```python
from build123d import *

# Parameters (mm, degrees)
SKETCH1_R           = 1.7526
BOSS_EXTRUDE1_DEPTH = 3


with BuildPart() as part:
    # Sketch1 → Boss-Extrude1 (new body)
    with BuildSketch(Plane.XY):
        with BuildLine():
            Line((-68.050090825, 31.75), (111.125, 31.75))
            Line((111.125, 31.75), (114.475, 31.75))
            Line((114.475, 31.75), (114.475, 19.05))
            Line((114.475, 19.05), (111.3, 19.05))
            Line((111.3, 19.05), (111.3, -6.35))
            Line((111.3, -6.35), (114.3, -6.35))
            Line((114.3, -6.35), (114.3, -18.229405084))
            Line((114.3, -18.229405084), (114.3, -19.870594916))
            Line((114.3, -19.870594916), (114.3, -31.75))
            Line((114.3, -31.75), (111.125, -31.75))
            Line((111.125, -31.75), (102.87, -31.75))
            Line((102.87, -31.75), (102.87, -34.75))
            Line((102.87, -34.75), (90.17, -34.75))
            Line((90.17, -34.75), (90.17, -31.75))
            Line((90.17, -31.75), (88.19515, -31.75))
            Line((88.19515, -31.75), (77.9653, -31.75))
            Line((77.9653, -31.75), (77.9653, -26.67))
            Line((77.9653, -26.67), (80.3275, -26.67))
            Line((80.3275, -26.67), (80.3275, -21.59))
            Line((80.3275, -21.59), (72.0725, -21.59))
            Line((72.0725, -21.59), (72.0725, -26.67))
            Line((72.0725, -26.67), (74.4347, -26.67))
            Line((74.4347, -26.67), (74.4347, -31.75))
            Line((74.4347, -31.75), (27.1653, -31.75))
            Line((27.1653, -31.75), (27.1653, -26.67))
            Line((27.1653, -26.67), (29.5275, -26.67))
            Line((29.5275, -26.67), (29.5275, -21.59))
            Line((29.5275, -21.59), (21.2725, -21.59))
            Line((21.2725, -21.59), (21.2725, -26.67))
            Line((21.2725, -26.67), (23.6347, -26.67))
            Line((23.6347, -26.67), (23.6347, -31.75))
            Line((23.6347, -31.75), (9.525, -31.75))
            Line((9.525, -31.75), (9.525, -34.75))
            Line((9.525, -34.75), (-9.525, -34.75))
            Line((-9.525, -34.75), (-9.525, -31.75))
            Line((-9.525, -31.75), (-23.6347, -31.75))
            Line((-23.6347, -31.75), (-23.6347, -26.67))
            Line((-23.6347, -26.67), (-21.2725, -26.67))
            Line((-21.2725, -26.67), (-21.2725, -21.59))
            Line((-21.2725, -21.59), (-29.5275, -21.59))
            Line((-29.5275, -21.59), (-29.5275, -26.67))
            Line((-29.5275, -26.67), (-27.1653, -26.67))
            Line((-27.1653, -26.67), (-27.1653, -31.75))
            Line((-27.1653, -31.75), (-41.275, -31.75))
            Line((-41.275, -31.75), (-41.275, -34.75))
            Line((-41.275, -34.75), (-60.325, -34.75))
            Line((-60.325, -34.75), (-60.325, -31.75))
            Line((-60.325, -31.75), (-74.4347, -31.75))
            Line((-74.4347, -31.75), (-74.4347, -26.67))
            Line((-74.4347, -26.67), (-72.0725, -26.67))
            Line((-72.0725, -26.67), (-72.0725, -21.59))
            Line((-72.0725, -21.59), (-80.3275, -21.59))
            Line((-80.3275, -21.59), (-80.3275, -26.67))
            Line((-80.3275, -26.67), (-77.9653, -26.67))
            Line((-77.9653, -26.67), (-77.9653, -31.75))
            Line((-77.9653, -31.75), (-114.3, -31.75))
            add(Edge.make_bspline(
                [(-114.3, -31.75), (-155.042938789, -12.240400658), (-94.548851624, -1.377525337), (-82.535055103, 31.754341042), (-68.050090825, 31.75)],
                knots=[0, 0, 0, 0, 0.655069171, 1, 1, 1, 1], degree=3))
        make_face()
        with Locations((112.395, -19.05)):
            Circle(SKETCH1_R, mode=Mode.SUBTRACT)
    extrude(amount=BOSS_EXTRUDE1_DEPTH)


solid = part.part
```
CAD build for the part. Positions are in the model's coordinates, mm. Coordinates: 2 decimals unless noted, no trailing zeros. Order: outer loops, then holes, each group sorted by start corner. A loop starts at its lowest first (then second) coordinate and runs counter-clockwise, first axis right, second up. Notation, with made-up numbers: (84, -14) -> (114, -14) arc R23 cw to (114, -2) -> close; hole circle Ø8 at (84, -12). An arc over 180 degrees is marked (long way). Use one line per item in the form item = value. Start each with the question number.
1) Drill centre lines: L1, parallel to Y at x = 27.5, z = 1.8; L2, parallel to X at y = -28, z = 1; L3, parallel to Y at x = 13, z = 1.9. Where is each one in solid material? Low to high. Write a range as [from, to].
2) Band-saw the part on A-A on x = 35. Give the cut face in (y, z), then the cut area to 4 significant figures.
3) Drop flat-ended pins along their axis: pin 1 (1.5 mm diameter, centred on y = -33, z = 1, fed in from -X) (3 decimals); pin 2 (1.2 mm diameter, centred on x = -73.5, z = 2, fed in from +Y); pin 3 (1.5 mm diameter, centred on y = -28.5, z = 1, fed in from +X). Give the stop position or say it passes through.
Entries:
q1.L1 = [-31.75, -26.67], [-21.59, 31.75]
q1.L2 = [-121.42, -77.97], [-74.43, -27.17], [-23.63, 23.63], [27.17, 74.43], [77.97, 114.3]
q1.L3 = [-31.75, 31.75]
q2.outline = (-31.75, 0) -> (31.75, 0) -> (31.75, 3) -> (-31.75, 3) -> close
q2.area = 190.5 mm2
q3.pin_1 = -60.325
q3.pin_2 = 31.27
q3.pin_3 = 114.3
